Input: dimensioned drawing with shaded views. Units: mm. Origin: part minimum x, y, z. A direction names the side the tool comes from. Round coordinates to 2 decimals unless told otherwise and drop trailing zeros. Write each loop counter-clockwise with the first axis right and the second up, starting at its lowest first coordinate (ties: lowest second). Pieces come first, ordered by that corner, then holes. Notation, with made-up numbers: M 16.5,-31.75 L 29.5,-31.75 A28 cw 29.5,7.25 Z; hole C 38,-14 d4. An arc over 180 degrees is marked long. Answer in a Markdown table with one row per item. Add a question column.
Item 1: Cut plane B-B on y = 17.5. Return loops of the section in (x, z), and give its area (3 significant figures).
Item 2: Cut plane C-C on z = 20. Return loops of the section in (x, y), and give its area (3 significant figures).
Item 3: Set-up query: the marked faces 4, 5, 6, 7 and 8. Return all of +Z, -Z, +X, -X, +Y, -Y with unobstructed straight access to the full face (end or side cutting, diameter ignored); none if empty.
Item 4: Cut plane D-D on y = 13.5. Return loops of the section in (x, z), and give its area (3 significant figures).
Item 5: Contact query for flat-ended pins moving along their axis: pin 1 (1.5 mm diameter, centred on y = 5.5, z = 15.5, fed in from -X); pin 2 (7 mm diameter, centred on y = 16, z = 7.5, fed in from +X); pin 3 (3.5 mm diameter, centred on x = 13, y = 25.5, fed in from -Z); pin 4 (4 mm diameter, centred on x = 11.5, y = 17.5, fed in from -Z) (1 decimal). Output: stop coordinate, or through.
Item 6: Material intervals for probe 1 along Y at (x, z) = (11.5, 26.15); probe 2 along Y at (x, z) = (11.5, 25.1); probe 3 along X at (y, z) = (26, 16.25), sorted ascending.
Item 7: Cut plane A-A on x = 13. Return loops of the section in (y, z).
Item 8: Mould query, pull axis Y, two halves, no side actions, for the marked faces 1, 2 and 3. Classes: released by +Y, released by -Y, zero draft, split by the parting line, or undercut.
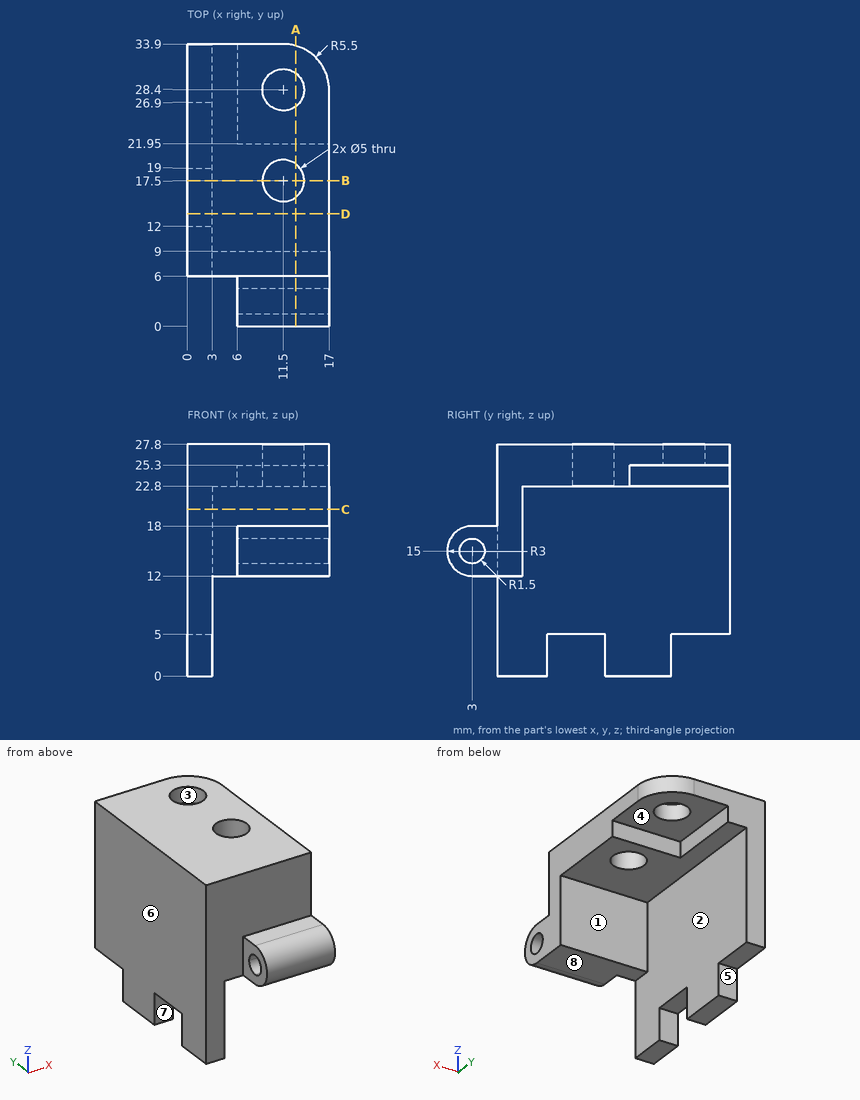
Results below:
| question | item | result |
|---|---|---|
| 1 | outline | M 0,5 L 3,5 L 3,22.8 L 9,22.8 L 9,27.8 L 0,27.8 Z; M 14,22.8 L 17,22.8 L 17,27.8 L 14,27.8 Z |
| 1 | area | 113 mm2 |
| 2 | outline | M 0,6 L 17,6 L 17,9 L 3,9 L 3,33.9 L 0,33.9 Z |
| 2 | area | 126 mm2 |
| 3 | face 4 | -Z, +X, +Y |
| 3 | face 5 | -Z, +X, -X, +Y |
| 3 | face 6 | +Z, -Z, -X, +Y, -Y |
| 3 | face 7 | -Z, +X, -X |
| 3 | face 8 | -Z, +X, +Y, -Y |
| 4 | outline | M 0,5 L 3,5 L 3,22.8 L 17,22.8 L 17,27.8 L 0,27.8 Z |
| 4 | area | 138 mm2 |
| 5 | pin 1 | x = 0 |
| 5 | pin 2 | x = 3 |
| 5 | pin 3 | z = 25.3 |
| 5 | pin 4 | through |
| 6 | probe 1 | 6 to 15, 20 to 25.9, 30.9 to 33.9 |
| 6 | probe 2 | 6 to 15, 20 to 21.95 |
| 6 | probe 3 | 0 to 3 |
| 7 | outline | M 3,12 L 9,12 L 9,22.8 L 15.5,22.8 L 15.5,27.8 L 6,27.8 L 6,18 L 3,18 A3 ccw Z; M 19.5,22.8 L 21.95,22.8 L 21.95,25.3 L 26.4,25.3 L 26.4,27.8 L 19.5,27.8 Z; M 30.4,25.3 L 33.69,25.3 L 33.69,27.8 L 30.4,27.8 Z; hole C 3,15 d3 |
| 8 | face 1 | released by +Y |
| 8 | face 2 | zero draft |
| 8 | face 3 | undercut |
